Check sheet for the modelled part. Datum: model origin and axes. Units: mm. A direction names the side the tool comes from. Give positions to 0.01 mm unless a question says otherwise; leave off trailing zeros. Order: outer loops, then holes, each group sorted by start corner. A loop starts at its lowest first (then second) coordinate and runs counter-clockwise, first axis right, second up. Notation, with made-up numbers: (-5.75, 10) -> (38.25, 10) arc R19 ccw to (38.25, 18) -> close; hole circle Ø2 at (57, 30). An arc over 180 degrees is marked (long way). Write each question's results on one line, items separated by ' | '.
from build123d import *

# Parameters (mm, degrees)
F0_R      = 17.018
F1_DEPTH  = 4
F4_R      = 2.5
F5_DEPTH  = 2
F7_R      = 1.905
F8_DEPTH  = 25.4
F9_R      = 13.9564544628
F9_R_2    = 1.905
F9_R_3    = 2.5
F10_DEPTH = 2.54


# Not quite as in the source:
# - the program builds the solid bodies; features that only make, move or delete a surface that nothing else refers to are left out


with BuildPart() as f1:
    # F0 (on Front) → F1 (new body)
    with BuildSketch(Plane.XZ):
        Circle(F0_R)
    extrude(amount=-F1_DEPTH)

    # F4 (on Front) → F5 (join)
    with BuildSketch(Plane.XZ):
        Circle(F4_R)
    extrude(amount=F5_DEPTH)

    # F7 (on face) → F8 (cut)
    with BuildSketch(Plane.XZ):
        with Locations((-7.4105341768, 7.4105341768)):
            Circle(F7_R)
        with Locations((0, 10.4800779372)):
            Circle(F7_R)
        with Locations((7.4105341768, 7.4105341768)):
            Circle(F7_R)
        with Locations((10.4800779372, 0)):
            Circle(F7_R)
        with Locations((7.4105341768, -7.4105341768)):
            Circle(F7_R)
        with Locations((0, -10.4800779372)):
            Circle(F7_R)
        with Locations((-7.4105341768, -7.4105341768)):
            Circle(F7_R)
        with Locations((-10.4800779372, 0)):
            Circle(F7_R)
    extrude(amount=-F8_DEPTH, mode=Mode.SUBTRACT)

    # F9 (on face) → F10 (cut)
    with BuildSketch(Plane.XZ):
        Circle(F9_R)
        with Locations((-7.4105341768, -7.4105341768)):
            Circle(F9_R_2, mode=Mode.SUBTRACT)
        with Locations((0, -10.4800779372)):
            Circle(F9_R_2, mode=Mode.SUBTRACT)
        with Locations((7.4105341768, -7.4105341768)):
            Circle(F9_R_2, mode=Mode.SUBTRACT)
        with Locations((-10.4800779372, 0)):
            Circle(F9_R_2, mode=Mode.SUBTRACT)
        with Locations((-7.4105341768, 7.4105341768)):
            Circle(F9_R_2, mode=Mode.SUBTRACT)
        Circle(F9_R_3, mode=Mode.SUBTRACT)
        with Locations((7.4105341768, 7.4105341768)):
            Circle(F9_R_2, mode=Mode.SUBTRACT)
        with Locations((10.4800779372, 0)):
            Circle(F9_R_2, mode=Mode.SUBTRACT)
        with Locations((0, 10.4800779372)):
            Circle(F9_R_2, mode=Mode.SUBTRACT)
    extrude(amount=-F10_DEPTH, mode=Mode.SUBTRACT)


solid = f1.part
1. Section check D-D on z = 11. Record the cut outline in (x, y).
Verdict:
outline: (-12.99, 0) -> (-8.59, 0) -> (-8.59, 2.54) -> (-1.83, 2.54) -> (-1.83, 4) -> (-12.99, 4) -> close; (1.83, 2.54) -> (8.59, 2.54) -> (8.59, 0) -> (12.99, 0) -> (12.99, 4) -> (1.83, 4) -> close
2. Section check C-C on y = 0.85. Record the cut outline in (x, z).
Verdict:
outline: circle Ø34.04 at (0, 0); circle Ø5 at (0, 0); hole circle Ø27.91 at (0, 0)
3. Section check B-B on z = 7. Record the cut outline in (x, y).
Verdict:
outline: (-15.51, 0) -> (-12.07, 0) -> (-12.07, 2.54) -> (-9.27, 2.54) -> (-9.27, 4) -> (-15.51, 4) -> close; (-5.55, 2.54) -> (5.55, 2.54) -> (5.55, 4) -> (-5.55, 4) -> close; (9.27, 2.54) -> (12.07, 2.54) -> (12.07, 0) -> (15.51, 0) -> (15.51, 4) -> (9.27, 4) -> close
4. Access from +Z, -Z, +X, -X, +Y, -Y to the whole of each face (thin tool, end or side, straight path). Record for faces 4 (the cylindrical face through (-7.66, 3.26, 9.3)), 5 (the cylindrical face through (-10.29, 1.25, 9.43)).
Verdict:
face 4: +Y, -Y | face 5: -Y
5. Section check A-A on x = 0. Record the cut outline in (y, z), then the cut area to 3 significant figures.
Verdict:
outline: (-2, -2.5) -> (2.54, -2.5) -> (2.54, -8.58) -> (4, -8.58) -> (4, 8.58) -> (2.54, 8.58) -> (2.54, 2.5) -> (-2, 2.5) -> close; (0, -17.02) -> (4, -17.02) -> (4, -12.39) -> (2.54, -12.39) -> (2.54, -13.96) -> (0, -13.96) -> close; (0, 13.96) -> (2.54, 13.96) -> (2.54, 12.39) -> (4, 12.39) -> (4, 17.02) -> (0, 17.02) -> close | area: 76.8 mm^2
6. Gauge pin test, flat ends, axial feed: pin 1 Ø6 at (x, z) = (-10.48, 0) entering from -Y; pin 2 Ø1 at (y, z) = (2.5, 1.5) entering from +X. Record the tip position at first contact, or that the pin passes through.
Verdict:
pin 1: stops at y = 2.54 | pin 2: stops at x = 16.99
7. Material ranges on probe 1 along Z at (x, y) = (-1, 1.9); probe 2 along Y at (x, z) = (4.5, -8); probe 3 along Y at (x, z) = (9, -14), recorded low to high. Write a range as from..to.
Verdict:
probe 1: z = -16.99..-13.92, -2.29..2.29, 13.92..16.99 | probe 2: y = 2.54..4 | probe 3: y = 0..4
8. Mould release check, pull along Z, two halves, no side actions. Record for faces 1 (the cylindrical face through (-2.215, 1.972, 16.873)), 2 (the cylindrical face through (12.24, 3.26, -0.73)), 3 (the flat face through (0, -2, 0)): +Z half, -Z half, draft (parallel to the pull), parting line (faces both ways), or undercut.
Verdict:
face 1: parting line | face 2: undercut | face 3: draft
